from build123d import *

# Parameters (mm, degrees)
SKETCH_4_R            = 72.55
EXTRUDE_297_DEPTH     = 70
SKETCH_8_R            = 62.55
SKETCH_8_R_2          = 58
CUT_EXTRUDE_406_DEPTH = 7
SKETCH_9_R            = 55
CUT_EXTRUDE_3_DEPTH   = 70


with BuildPart() as part:
    # 草圖4 → Extrude 297 (new body)
    with BuildSketch(Plane(origin=(0, 0, 0), x_dir=(1, 0, 0), z_dir=(0, 1, 0))):
        with Locations(Location((0, 0, 0), (0, 0, 270))):
            Circle(SKETCH_4_R)
    extrude(amount=EXTRUDE_297_DEPTH)

    # 草圖8 → Cut-Extrude 406 (cut)
    with BuildSketch(Plane(origin=(0, 70, 0), x_dir=(1, 0, 0), z_dir=(0, 1, 0))):
        with Locations(Location((0, 0, 0), (0, 0, 270))):
            Circle(SKETCH_8_R)
        with Locations(Location((0, 0, 0), (0, 0, 270))):
            Circle(SKETCH_8_R_2, mode=Mode.SUBTRACT)
    extrude(amount=-CUT_EXTRUDE_406_DEPTH, mode=Mode.SUBTRACT)

    # 草圖9 → 除料-伸長3 (cut)
    with BuildSketch(Plane(origin=(0, 70, 0), x_dir=(1, 0, 0), z_dir=(0, 1, 0))):
        with Locations(Location((0, 0, 0), (0, 0, 270))):
            Circle(SKETCH_9_R)
    extrude(amount=-CUT_EXTRUDE_3_DEPTH, mode=Mode.SUBTRACT)


solid = part.part
Can you work these out from the model? Positions are in its coordinate system, mm. A direction names the side the tool comes from. Coordinates: 2 decimals unless noted, no trailing zeros. Write each loop counter-clockwise with the first axis right and the second up, starting at its lowest first coordinate (ties: lowest second). Pieces come first, ordered by that corner, then holes. Notation, with made-up numbers: (12.25, 66.5) -> (20.25, 66.5) arc R11 ccw to (20.25, 75.5) -> close; hole circle Ø11 at (18.25, -28). An arc over 180 degrees is marked (long way). Write each question's results on one line, items separated by ' | '. Start each with the question number.
Q1. Imagine slicing it at A-A (x = 0). Write out the boundary of the cut face in (y, z), then the cut area to 3 significant figures.
Q2. Imagine slicing it at B-B (z = 0). Write out the boundary of the cut face in (x, y).
Q3. I'm going to push flat-ended pins straight in: pin 1 (5 mm diameter, centred on x = -9, y = 23.5, fed in from -Z); pin 2 (1 mm diameter, centred on y = 61, z = -49.5, fed in from +X); pin 3 (1.5 mm diameter, centred on x = 41, z = -33, fed in from -Y); pin 4 (4 mm diameter, centred on x = 52.5, y = 10, fed in from +Z). Where does each tip first touch, or does it pass through?
Q4. If I drill on probe 1 along X at (y, z) = (14, 0); probe 2 along X at (y, z) = (40, 48.5); probe 3 along Z at (x, y) = (-28, 46), over which ranges is the centre line in solid material (lowest first)?
Q5. We'd pull the mould along Z, two halves only. Please class faces 1 (the face through (-70.825, 34.51, -15.727)), 2 (the face through (54, 70, 32)), 3 (the face through (-22.21, 66.55, 53.58)): +Z half, -Z half, draft (parallel to the pull), parting line (faces both ways), or undercut.
Q6. Imagine slicing it at C-C (y = 6). Write out the boundary of the cut face in (x, z).
Q7. On a 3-axis mill with a long thin cutter (end or side, diameter ignored), from which of +Z, -Z, +X, -X, +Y, -Y can I reach the whole of each face in a straight line? I mean faces 4 (the face through (-48.794, 35.49, 25.379)), 5 (the face through (-38.06, 66.55, -49.64)). Say none if no direction works.
Taken from the geometry:
1) outline: (0, -72.55) -> (70, -72.55) -> (70, -62.55) -> (63, -62.55) -> (63, -58) -> (70, -58) -> (70, -55) -> (0, -55) -> close; (0, 55) -> (70, 55) -> (70, 58) -> (63, 58) -> (63, 62.55) -> (70, 62.55) -> (70, 72.55) -> (0, 72.55) -> close | area: 2,390 mm^2
2) outline: (-72.55, 0) -> (-55, 0) -> (-55, 70) -> (-58, 70) -> (-58, 63) -> (-62.55, 63) -> (-62.55, 70) -> (-72.55, 70) -> close; (55, 0) -> (72.55, 0) -> (72.55, 70) -> (62.55, 70) -> (62.55, 63) -> (58, 63) -> (58, 70) -> (55, 70) -> close
3) pin 1: stops at z = -72.26 | pin 2: stops at x = 53.5 | pin 3: passes through | pin 4: stops at z = 52.09
4) probe 1: x = -72.55 to -55, 55 to 72.55 | probe 2: x = -53.96 to -25.94, 25.94 to 53.96 | probe 3: z = -66.93 to -47.34, 47.34 to 66.93
5) face 1: parting line | face 2: draft | face 3: undercut
6) outline: circle Ø145.1 at (0, 0); hole circle Ø110 at (0, 0)
7) face 4: +Y, -Y | face 5: +Y
